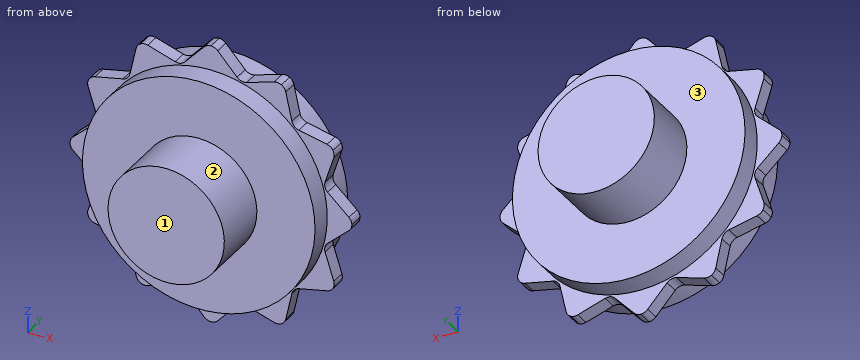
```python
from build123d import *

# Parameters (mm, degrees)
SKETCH1_R           = 6.35
BOSS_EXTRUDE1_DEPTH = 19.05
BOSS_EXTRUDE2_START = 6.35
SKETCH2_R           = 12.7
BOSS_EXTRUDE2_DEPTH = 6.35
BOSS_EXTRUDE3_DEPTH = 0.79375
CIRPATTERN1_COUNT   = 12


with BuildPart() as part:
    # Sketch1 → Boss-Extrude1 (new body)
    with BuildSketch(Plane(origin=(0, 0, 0), x_dir=(1, 0, 0), z_dir=(0, 1, 0))):
        with Locations(Location((0, 0, 0), (0, 0, 270))):
            Circle(SKETCH1_R)
    extrude(amount=BOSS_EXTRUDE1_DEPTH)

    # Sketch2 → Boss-Extrude2 (add)
    with BuildSketch(Plane(origin=(0, 0, 0), x_dir=(1, 0, 0), z_dir=(0, 1, 0)).offset(BOSS_EXTRUDE2_START)):
        with Locations(Location((0, 0, 0), (0, 0, 270))):
            Circle(SKETCH2_R)
    extrude(amount=BOSS_EXTRUDE2_DEPTH)

    # Sketch3 → Boss-Extrude3 (add, symmetric)
    with BuildSketch(Plane(origin=(0, 9.525, 0), x_dir=(1, 0, 0), z_dir=(0, 1, 0))):
        with BuildLine():
            Line((-6.891666757, -13.415120246), (-3.89786608, -12.461780366))
            ThreePointArc((-3.89786608, -12.461780366), (-3.335621729, -12.448709767), (-2.855239137, -12.741151414))
            Line((-2.855239137, -12.741151414), (-0.739201637, -15.063668306))
            ThreePointArc((-0.739201637, -15.063668306), (-0.404051866, -15.304920203), (0, -15.390184127))
            Line((0, -15.390184127), (0, -12.7))
            Line((0, -12.7), (-6.35, -10.998522628))
            Line((-6.35, -10.998522628), (-7.695092063, -13.328290423))
            ThreePointArc((-7.695092063, -13.328290423), (-7.302540921, -13.456475632), (-6.891666757, -13.415120246))
        make_face()
    boss_extrude3 = extrude(amount=BOSS_EXTRUDE3_DEPTH, both=True)

    # CirPattern1: Boss-Extrude3 ×12 about axis
    cirpattern1_axis = Axis((0, 0, 0), (0, 1, 0))
    for i in range(1, CIRPATTERN1_COUNT):
        add(boss_extrude3.rotate(cirpattern1_axis, i * 360 / CIRPATTERN1_COUNT))


solid = part.part
```
Build history of the part. All positions in model axes, mm. Face numbers are marked on the shaded views. A direction names the side the tool comes from. Give positions to 0.01 mm unless a question says otherwise; leave off trailing zeros. Order: outer loops, then holes, each group sorted by start corner. A loop starts at its lowest first (then second) coordinate and runs counter-clockwise, first axis right, second up. Notation, with made-up numbers: M 55,-11 L 62,-11 A15 cw 62,-7 Z; hole C -16,0 d1. An arc over 180 degrees is marked long. Write item = value, one per line. Start each with the question number.
(1) Slice it at C-C on x = -12. Write the cut outline in (y, z).
(2) Slice it at A-A on x = -3.5. Write the cut outline in (y, z), plus the area to 3 significant figures.
(3) Which spindle directions (+Z, -Z, +X, -X, +Y, -Y) get a long thin tool onto all of the face, cutting with end or side? Do the marked faces 1, 2 and 3. Say none if no direction does.
(4) Probe L1, parallel to Y at x = -9, z = -2.5; L2, parallel to Y at x = 13, z = 7; L3, parallel to X at y = 9.5, z = -1. List the from-to ranges inside material, lowest first. Write a range as [from, to].
(5) Slice it at B-B on y = 13.75. Write the cut outline in (x, z).
(6) Pin check, flat tips, straight feed: pin 1 Ø3 at (y, z) = (8.5, -2.5) entering from +X; pin 2 Ø3 at (x, z) = (1, 9.5) entering from +Y; pin 3 Ø8 at (x, z) = (-10, -6) entering from -Y. Stop position of each tip, or through.
(7) Slice it at D-D on y = 11.75. Write the cut outline in (x, z).
Responses:
q1.outline = M 6.35,-4.16 L 8.73,-4.16 L 8.73,-8.32 L 10.32,-8.32 L 10.32,-4.16 L 12.7,-4.16 L 12.7,4.16 L 10.32,4.16 L 10.32,8.32 L 8.73,8.32 L 8.73,4.16 L 6.35,4.16 Z
q2.outline = M 0,-5.3 L 6.35,-5.3 L 6.35,-12.21 L 8.73,-12.21 L 8.73,-12.42 L 10.32,-12.42 L 10.32,-12.21 L 12.7,-12.21 L 12.7,-5.3 L 19.05,-5.3 L 19.05,5.3 L 12.7,5.3 L 12.7,12.21 L 10.32,12.21 L 10.32,12.42 L 8.73,12.42 L 8.73,12.21 L 6.35,12.21 L 6.35,5.3 L 0,5.3 Z
q2.area = 290 mm2
q3.face_1 = +Z, -Z, +X, -X, -Y
q3.face_2 = -Y
q3.face_3 = +Y
q4.L1 = [6.35, 12.7]
q4.L2 = [8.73, 10.32]
q4.L3 = [-14.78, 14.78]
q5.outline = C 0,0 d12.7
q6.pin_1 = 14.76
q6.pin_2 = 12.7
q6.pin_3 = 6.35
q7.outline = C 0,0 d25.4
